Answer from the drawing. Dimensions are ordinates in mm from the lowest x, y and z of the part. Round coordinates to 2 decimals unless told otherwise and drop trailing zeros. Write each loop counter-clockwise with the first axis right and the second up, starting at its lowest first coordinate (ties: lowest second). Pieces come first, ordered by that corner, then holes. Notation, with made-up numbers: (-27, -12.75) - (16, -12.75) arc R29 ccw to (16, 19.25) - close; hole circle Ø6 at (83, 40.5). An arc over 180 degrees is marked (long way). Answer as a JSON object with one key per item and string values.
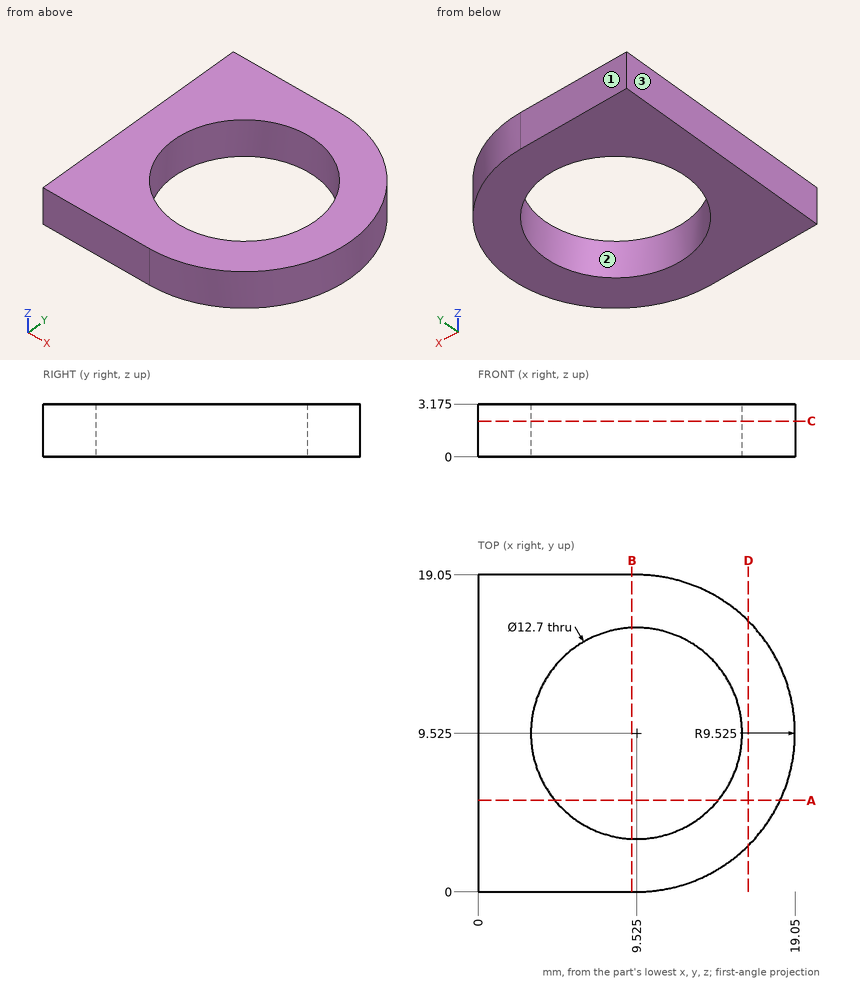
Item 1: A cutting plane is placed at B-B (x = 9.25). Write down the section's boundary in (y, z) (3 decimals).
Results found:
{"outline": "(0, 0) - (3.181, 0) - (3.181, 3.175) - (0, 3.175) - close; (15.869, 0) - (19.05, 0) - (19.05, 3.175) - (15.869, 3.175) - close"}
Item 2: Consider line 1 along Y through (x, z) = (9.5, 2); line 2 along Y through (x, z) = (7.5, 2.7). Determine where each line is inside the solid, lowest interval first.
Results found:
{"line 1": "0 to 3.18, 15.87 to 19.05", "line 2": "0 to 3.51, 15.54 to 19.05"}
Item 3: A cutting plane is placed at A-A (y = 5.5). Write down the section's boundary in (x, z) (3 decimals).
Results found:
{"outline": "(0, 0) - (4.614, 0) - (4.614, 3.175) - (0, 3.175) - close; (14.436, 0) - (18.158, 0) - (18.158, 3.175) - (14.436, 3.175) - close"}
Item 4: Each of these flat-tipped pins is pushed along its axis until it touches: P1, Ø1.5, axis at x = 13.5, z = 0.5, coming from the -Y side; P2, Ø1.5, axis at x = 9.5, y = 3.5, coming from the -Z side. Where does it stop, or does it pass through?
Results found:
{"P1": "y = 0.56", "P2": "z = 0"}
Item 5: A cutting plane is placed at C-C (z = 2.15). Write down the section's boundary in (x, y) (3 decimals).
Results found:
{"outline": "(0, 0) - (9.525, 0) arc R9.525 ccw to (9.525, 19.05) - (0, 19.05) - close; hole circle Ø12.7 at (9.525, 9.525)"}
Item 6: Determine the mould class of the marked faces 1, 2 and 3 for opening direction Y: pulls with the +Y half, pulls with the -Y half, needs draft (parallel to the pull), parting line crosses it, or undercut.
Results found:
{"face 1": "pulls with the +Y half", "face 2": "undercut", "face 3": "needs draft"}
Item 7: A cutting plane is placed at D-D (x = 16.25). Write down the section's boundary in (y, z) (3 decimals), and give its area (3 significant figures).
Results found:
{"outline": "(2.78, 0) - (16.27, 0) - (16.27, 3.175) - (2.78, 3.175) - close", "area": "42.8 mm²"}
